Geometry: final body of the model. Coordinates: model frame, mm. Face numbers are marked on the shaded views. A direction names the side the tool comes from. Round coordinates to 2 decimals unless told otherwise and drop trailing zeros. Write each loop counter-clockwise with the first axis right and the second up, starting at its lowest first coordinate (ties: lowest second). Pieces come first, ordered by that corner, then holes. Notation, with made-up numbers: (45.25, 70) -> (80.25, 70) arc R33 cw to (80.25, 106) -> close; hole circle Ø1 at (65.5, 78). An arc over 180 degrees is marked (long way). Use one line per item in the form item = value. Start each with the question number.
1. Cut plane C-C, the plane x = 16.75. Return the cut outline in (y, z).
2. Cut plane A-A, the plane y = 21.5. Return the cut outline in (x, z).
3. Reachability of the marked faces 1, 2, 3 and 4 from +Z, -Z, +X, -X, +Y, -Y: full face, straight path, thin tool, end or side. Return the list, or none.
4. Line query: L1, parallel to Z at x = 4.5, y = 14.5; L2, parallel to Z at x = 15.75, y = 8; L3, parallel to X at y = 2.25, z = 12.75. Output: solid intervals per line, ascending.
5. Draft query along X for the marked faces 5, 6, 7 and 8. Return one class per face: pulls with the +X half, pulls with the -X half, needs draft (parallel to the pull), parting line crosses it, or undercut.
6. Cut plane B-B, the plane z = 13.25. Return the cut outline in (x, y), plus the area to 3 significant figures.
7. Pin query (flat end, axial travel): pin 1 Ø11 at (x, z) = (18.5, 15) entering from +Y; pin 2 Ø4 at (y, z) = (21, 10.5) entering from +X. Return the tip coordinate at first contact, or that it passes through.
8. Cut plane D-D, the plane y = 2.5. Return the cut outline in (x, z).
```python
from build123d import *

# Parameters (mm, degrees)
BOSS_EXTRUDE1_DEPTH = 28
BOSS_EXTRUDE2_DEPTH = 3
BOSS_EXTRUDE3_DEPTH = 3
SKETCH4_W           = 6.4
SKETCH4_H           = 12
CUT_EXTRUDE1_DEPTH  = 5
SKETCH5_W           = 12
SKETCH5_H           = 6.4
CUT_EXTRUDE2_DEPTH  = 5


with BuildPart() as part:
    # Sketch1 → Boss-Extrude1 (new body)
    with BuildSketch(Plane.XY):
        Polygon((5, 5), (27, 5), (27, 0), (0, 0), (0, 27), (5, 27), align=None)
    extrude(amount=BOSS_EXTRUDE1_DEPTH)

    # Sketch1_3 → Boss-Extrude2 (add)
    with BuildSketch(Plane.XY):
        Polygon((5, 27), (5, 5), (27, 5), align=None)
    extrude(amount=BOSS_EXTRUDE2_DEPTH)

    # Sketch3 → Boss-Extrude3 (add)
    with BuildSketch(Plane.XY.offset(28)):
        Polygon((5, 27), (27, 5), (5, 5), align=None)
    extrude(amount=-BOSS_EXTRUDE3_DEPTH)

    # Sketch4 → Cut-Extrude1 (cut)
    with BuildSketch(Plane(origin=(5, 0, 0), x_dir=(0, 0, -1), z_dir=(1, 0, 0))):
        with Locations((-14, 16)):
            Rectangle(SKETCH4_W, SKETCH4_H)
    extrude(amount=-CUT_EXTRUDE1_DEPTH, mode=Mode.SUBTRACT)

    # Sketch5 → Cut-Extrude2 (cut)
    with BuildSketch(Plane(origin=(0, 5, 0), x_dir=(1, 0, 0), z_dir=(0, 1, 0))):
        with Locations((16, -14)):
            Rectangle(SKETCH5_W, SKETCH5_H)
    extrude(amount=-CUT_EXTRUDE2_DEPTH, mode=Mode.SUBTRACT)


solid = part.part
```
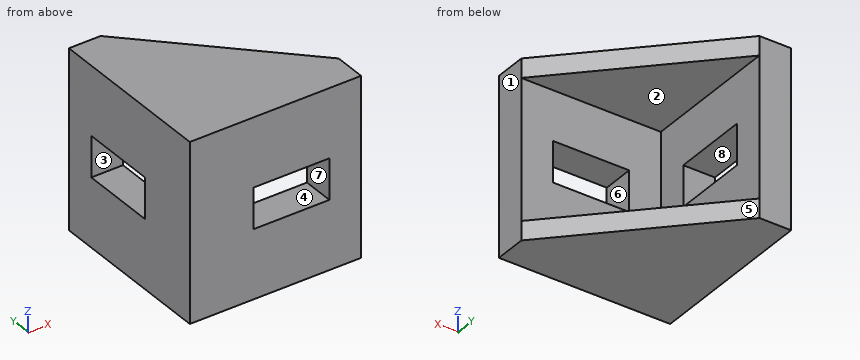
Outcome:
q1.outline = (0, 0) -> (15.25, 0) -> (15.25, 3) -> (5, 3) -> (5, 10.8) -> (0, 10.8) -> close; (0, 17.2) -> (5, 17.2) -> (5, 25) -> (15.25, 25) -> (15.25, 28) -> (0, 28) -> close
q2.outline = (0, 0) -> (10.5, 0) -> (10.5, 3) -> (5, 3) -> (5, 10.8) -> (0, 10.8) -> close; (0, 17.2) -> (5, 17.2) -> (5, 25) -> (10.5, 25) -> (10.5, 28) -> (0, 28) -> close
q3.face_1 = +Z, -Z, +X, +Y, -Y
q3.face_2 = +X, +Y
q3.face_3 = +X, -X
q3.face_4 = +Y, -Y
q4.L1 = 0 to 10.8, 17.2 to 28
q4.L2 = 0 to 3, 25 to 28
q4.L3 = 0 to 10, 22 to 27
q5.face_5 = pulls with the +X half
q5.face_6 = undercut
q5.face_7 = undercut
q5.face_8 = needs draft
q6.outline = (0, 0) -> (10, 0) -> (10, 5) -> (5, 5) -> (5, 10) -> (0, 10) -> close; (0, 22) -> (5, 22) -> (5, 27) -> (0, 27) -> close; (22, 0) -> (27, 0) -> (27, 5) -> (22, 5) -> close
q6.area = 125 mm^2
q7.pin_1 = 5
q7.pin_2 = 5
q8.outline = (0, 0) -> (27, 0) -> (27, 28) -> (0, 28) -> close; hole (10, 10.8) -> (22, 10.8) -> (22, 17.2) -> (10, 17.2) -> close
